from build123d import *

# Parameters (mm, degrees)
SKETCH1_R               = 18.5
BOSS_EXTRUDE1_DEPTH     = 22.5
SKETCH2_R               = 1.6
CUT_EXTRUDE1_DEPTH      = 3.5
SKETCH3_R               = 3
BOSS_EXTRUDE2_DEPTH     = 36.3
SKETCH3_3_R             = 6
SKETCH3_3_R_2           = 3
BOSS_EXTRUDE3_DEPTH     = 6.3
SKETCH4_R               = 14.5
BOSS_EXTRUDE4_DEPTH     = 37.8
SKETCH5_R               = 5
BOSS_EXTRUDE5_DEPTH     = 3
SKETCH6_R               = 1
BOSS_EXTRUDE6_DEPTH     = 9
SKETCH7_W               = 0.5
SKETCH7_H               = 3
BOSS_EXTRUDE7_DEPTH     = 6.5
CUT_EXTRUDE2_DEPTH      = 0.5
FILLET1_R               = 0.5
CHAMFER1_SIZE           = 0.2
SKETCH9_R               = 1.6
CUT_EXTRUDE3_DEPTH      = 12.5
CUT_EXTRUDE3_DEPTH_BACK = 26.5
SCALE1_SCALE            = 0.6757


with BuildPart() as part:
    # Sketch1 → Boss-Extrude1 (new body)
    with BuildSketch(Plane.XY):
        Circle(SKETCH1_R)
    extrude(amount=BOSS_EXTRUDE1_DEPTH)

    # Sketch2 → Cut-Extrude1 (cut)
    with BuildSketch(Plane.XY.offset(22.5)):
        with Locations((-7.75, 13.423393759)):
            Circle(SKETCH2_R)
        with Locations((7.75, 13.423393759)):
            Circle(SKETCH2_R)
        with Locations((-15.5, 0)):
            Circle(SKETCH2_R)
        with Locations((-7.75, -13.423393759)):
            Circle(SKETCH2_R)
        with Locations((7.75, -13.423393759)):
            Circle(SKETCH2_R)
        with Locations((15.5, 0)):
            Circle(SKETCH2_R)
    extrude(amount=-CUT_EXTRUDE1_DEPTH, mode=Mode.SUBTRACT)

    # Sketch3 → Boss-Extrude2 (add)
    with BuildSketch(Plane.XY.offset(22.5)):
        with Locations((0, 7)):
            Circle(SKETCH3_R)
    extrude(amount=BOSS_EXTRUDE2_DEPTH)

    # Sketch3<3> → Boss-Extrude3 (add)
    with BuildSketch(Plane.XY.offset(22.5)):
        with Locations((0, 7)):
            Circle(SKETCH3_3_R)
        with Locations((0, 7)):
            Circle(SKETCH3_3_R_2, mode=Mode.SUBTRACT)
    extrude(amount=BOSS_EXTRUDE3_DEPTH)

    # Sketch4 → Boss-Extrude4 (add)
    with BuildSketch(Plane(origin=(0, 0, 0), x_dir=(-1, 0, 0), z_dir=(0, 0, -1))):
        Circle(SKETCH4_R)
    extrude(amount=BOSS_EXTRUDE4_DEPTH)

    # Sketch5 → Boss-Extrude5 (add)
    with BuildSketch(Plane(origin=(0, 0, -37.8), x_dir=(-1, 0, 0), z_dir=(0, 0, -1))):
        Circle(SKETCH5_R)
    extrude(amount=BOSS_EXTRUDE5_DEPTH)

    # Sketch6 → Boss-Extrude6 (add)
    with BuildSketch(Plane(origin=(0, 0, -40.8), x_dir=(-1, 0, 0), z_dir=(0, 0, -1))):
        Circle(SKETCH6_R)
    extrude(amount=BOSS_EXTRUDE6_DEPTH)

    # Sketch7 → Boss-Extrude7 (add)
    with BuildSketch(Plane(origin=(0, 0, -37.8), x_dir=(-1, 0, 0), z_dir=(0, 0, -1))):
        with Locations((-11.75, 0)):
            Rectangle(SKETCH7_W, SKETCH7_H)
        with Locations((11.75, 0)):
            Rectangle(SKETCH7_W, SKETCH7_H)
    extrude(amount=BOSS_EXTRUDE7_DEPTH)

    # Sketch8 → Cut-Extrude2 (cut)
    with BuildSketch(Plane(origin=(12, 0, 0), x_dir=(0, 0, -1), z_dir=(1, 0, 0))):
        with BuildLine():
            Line((42.865122037, -0.320114275), (41.665122037, -0.320114275))
            ThreePointArc((41.665122037, -0.320114275), (41.345007763, 0), (41.665122037, 0.320114275))
            Line((41.665122037, 0.320114275), (42.865122037, 0.320114275))
            ThreePointArc((42.865122037, 0.320114275), (43.185236312, 0), (42.865122037, -0.320114275))
        make_face()
    cut_extrude2 = extrude(amount=-CUT_EXTRUDE2_DEPTH, mode=Mode.SUBTRACT)

    # Mirror2: Cut-Extrude2 across plane
    add(cut_extrude2.mirror(Plane(origin=(0, 0, 0), x_dir=(0, 0, 1), z_dir=(1, 0, 0))), mode=Mode.SUBTRACT)

    # Fillet1
    fillet1_edges = [part.edges().sort_by_distance(p)[0] for p in [
        (11.75, -1.5, -44.3),
        (11.75, 1.5, -44.3),
        (-11.75, 1.5, -44.3),
        (-11.75, -1.5, -44.3),
    ]]
    fillet(fillet1_edges, radius=FILLET1_R)

    # Chamfer1
    chamfer1_edges = [part.edges().sort_by_distance(p)[0] for p in [
        (-3, 7, 58.8),
        (-6, 7, 28.8),
        (-18.5, 0, 22.5),
    ]]
    chamfer(chamfer1_edges, length=CHAMFER1_SIZE)

    # Sketch9 → Cut-Extrude3 (cut, two sides)
    with BuildSketch(Plane(origin=(0, 7, 0), x_dir=(1, 0, 0), z_dir=(0, 1, 0))) as cut_extrude3_sk:
        with Locations((0, -50.8)):
            Circle(SKETCH9_R)
    extrude(amount=CUT_EXTRUDE3_DEPTH, mode=Mode.SUBTRACT)
    extrude(cut_extrude3_sk.sketch, amount=-CUT_EXTRUDE3_DEPTH_BACK, mode=Mode.SUBTRACT)


with BuildPart() as part_1:
    # Scale1: scaled about (3.1e-08, 0.208571854, -3.181081733)
    add(part.part.scale(SCALE1_SCALE).moved(Location((1e-08, 0.067639852, -1.031624806))))


solid = part_1.part
For this review, take the finished solid that the model builds, in its own axes (mm). A direction names the side the tool comes from. Round coordinates to 2 decimals unless told otherwise and drop trailing zeros. Write each loop counter-clockwise with the first axis right and the second up, starting at its lowest first coordinate (ties: lowest second). Pieces come first, ordered by that corner, then holes. Notation, with made-up numbers: (-21.5, 56) -> (20.5, 56) arc R26 cw to (20.5, 74) -> close; hole circle Ø4 at (6, -1). An arc over 180 degrees is marked (long way). Use CSV: the item, a comma, the result in double quotes.
(1) Clearance check with flat-ended pins moving along their axes: P1, Ø0.6, axis at x = 5.5, y = 9, coming from the +Z side; P2, Ø2.5, axis at x = 5.5, y = -9.5, coming from the +Z side; P3, Ø2.5, axis at x = 5.24, y = 9.14, coming from the -Z side; P4, Ø1.9, axis at x = 0, z = 33.29, coming from the -Y side. State where each tip first meets the part, or that it passes through.
Computed values:
P1,"z = 11.81"
P2,"z = 14.17"
P3,"z = -26.57"
P4,"through"
(2) Consider section B-B, the plane z = 22. Give the boundary of the cut face in (x, y), plus the area to 3 significant figures.
Computed values:
outline,"circle Ø4.05 at (0, 4.8)"
area,"12.9 mm²"
(3) To check wall thickness, follow L1, parallel to Z at x = 0, y = 4.3; L2, parallel to Z at x = -6.75, y = -5.5; L3, parallel to Z at x = 5, y = -9. State the ranges of each line that lie inside material, in increasing order. Write a range as [from, to].
Computed values:
L1,"[-26.57, 32.21], [34.38, 38.7]"
L2,"[-26.57, 14.17]"
L3,"[-1.03, 11.81]"
(4) Consider section C-C, the plane z = -16. Give the boundary of the cut face in (x, y).
Computed values:
outline,"circle Ø19.6 at (0, 0.07)"
(5) For faces 1 (the face through (7.771, 0.1, -28.7)), 2 (the face through (-4, 0, -26.573)), 3 (the face through (-5, -9, 11.807)), 4 (the face through (8.108, 0.1, -28.7)), list the 3-axis set-ups (+Z, -Z, +X, -X, +Y, -Y) from which the entire face can be reached by the end or side of a thin tool; tool diameter is ignored.
Computed values:
face 1,"-Z, +Y, -Y"
face 2,"-Z"
face 3,"+Z"
face 4,"-Z, +X, +Y, -Y"
(6) Draft analysis for pull direction X (two halves, no side actions). For faces 5 (the face through (-8.108, 0.1, -28.7)), 6 (the face through (-7.771, 0.1, -28.7)), 7 (the face through (0, 5, 38.7)), state which applies: +X half, -X half, draft (parallel to the pull), parting line (faces both ways), or undercut.
Computed values:
face 5,"-X half"
face 6,"undercut"
face 7,"draft"
